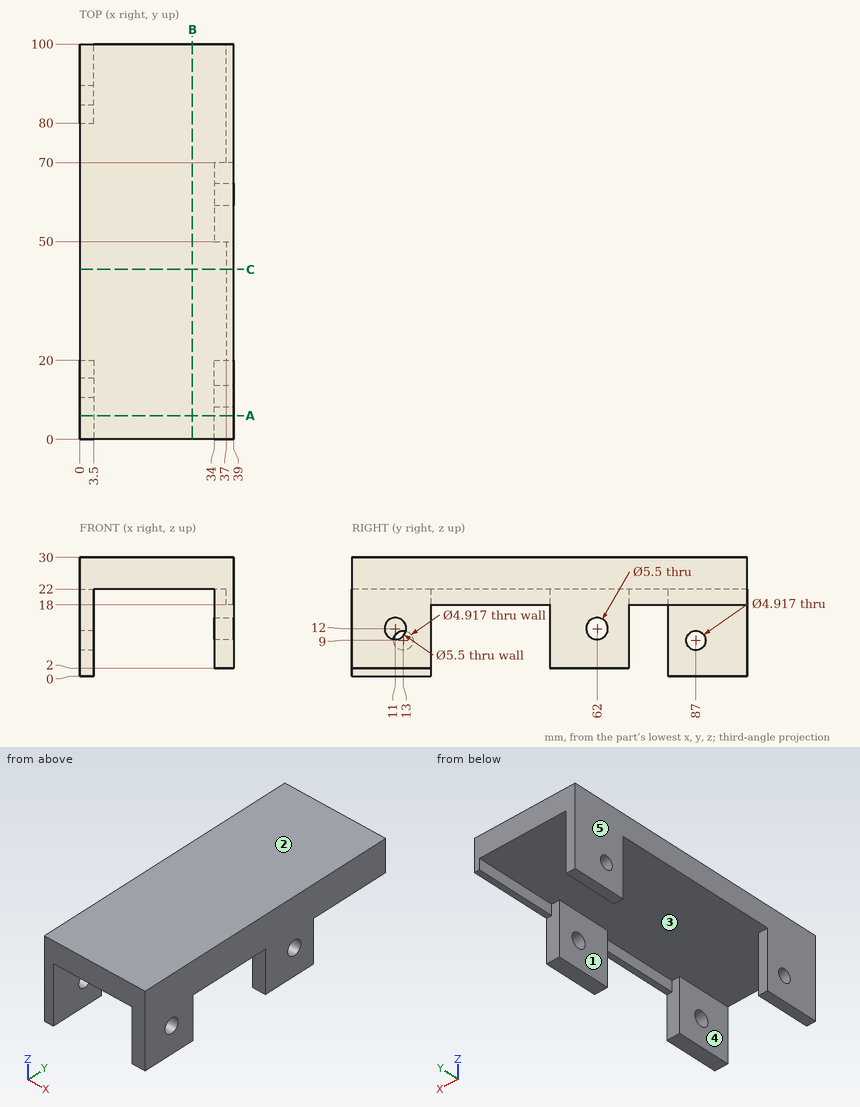
Source: three-view drawing plus pictorial views. Frame: mm from the lowest corner of the part. A direction names the side the tool comes from. Coordinates: 2 decimals unless noted, no trailing zeros. Loops run counter-clockwise (first coordinate to the right, second up) from the corner with the lowest first, then second, coordinate; pieces in that order, holes last. Notation, with made-up numbers: (-38.5, -14) - (-0.5, -14) arc R12 ccw to (-0.5, -6) - close; hole circle Ø3 at (29, 34.5). An arc over 180 degrees is marked (long way). Answer in a Markdown table with one row per item. Add a question column.
Item 1: Section query A-A on y = 6. Return the cut outline in (x, z), then the cut area to 3 significant figures.
Item 2: Access query for the marked faces 4 and 5. Directions: +Z, -Z, +X, -X, +Y, -Y. A direction counts if a zero-diameter tool reaches every point of the face in a straight line with its end or side. Return the directions, or none.
Item 3: Line query: line 1 along Y through (x, z) = (1.5, 9); line 2 along Z through (x, y) = (2.6, 13); line 3 along X through (y, z) = (19, 5.25). Output: solid intervals per line, ascending. Write a range as [from, to].
Item 4: Section query C-C on y = 43. Return the cut outline in (x, z).
Item 5: Contact query for flat-ended pins moving along their axis: P1, Ø1.6, axis at x = 38, y = 87, coming from the -Z side; P2, Ø3, axis at y = 39.5, z = 19, coming from the -X side; P3, Ø1.5, axis at x = 36.5, z = 11, coming from the +Y side; P4, Ø1, axis at y = 18, z = 13.5, coming from the -X side. Output: stop coordinate, or through.
Item 6: Section query B-B on x = 28.5. Return the cut outline in (y, z).
Item 7: Mould query, pull axis X, two halves, no side actions, for the marked faces 1, 2 and 3. Classes: released by +X, released by -X, zero draft, split by the parting line, or undercut.
Recorded:
| question | item | result |
|---|---|---|
| 1 | outline | (0, 0) - (3.5, 0) - (3.5, 22) - (34, 22) - (34, 2) - (39, 2) - (39, 30) - (0, 30) - close |
| 1 | area | 489 mm^2 |
| 2 | face 4 | -Z, +Y, -Y |
| 2 | face 5 | +Z, -Z, -X, +Y, -Y |
| 3 | line 1 | [0, 10.54], [15.46, 20], [80, 84.54], [89.46, 100] |
| 3 | line 2 | [0, 6.54], [11.46, 30] |
| 3 | line 3 | [0, 3.5], [34, 39] |
| 4 | outline | (0, 22) - (37, 22) - (37, 18) - (39, 18) - (39, 30) - (0, 30) - close |
| 5 | P1 | z = 18 |
| 5 | P2 | x = 37 |
| 5 | P3 | y = 70 |
| 5 | P4 | x = 0 |
| 6 | outline | (0, 22) - (100, 22) - (100, 30) - (0, 30) - close |
| 7 | face 1 | released by -X |
| 7 | face 2 | zero draft |
| 7 | face 3 | undercut |
